from build123d import *

# Parameters (mm, degrees)
EXTRUDE_1_DEPTH = 95
SKETCH_3_W      = 60
SKETCH_3_H      = 60
EXTRUDE_3_DEPTH = 8.5
SKETCH_5_R      = 25
EXTRUDE_5_DEPTH = 3
SKETCH_7_R      = 7
EXTRUDE_6_DEPTH = 25
CHAMFER_1_SIZE  = 3


with BuildPart() as part:
    # 草图1 → 凸台-拉伸1 (new body)
    with BuildSketch(Plane.XY):
        with BuildLine():
            Line((7.5, 0), (52.5, 0))
            ThreePointArc((52.5, 0), (54.696699141, -5.303300859), (60, -7.5))
            Line((60, -7.5), (60, -52.5))
            ThreePointArc((60, -52.5), (54.696699141, -54.696699141), (52.5, -60))
            Line((52.5, -60), (7.5, -60))
            ThreePointArc((7.5, -60), (5.303300859, -54.696699141), (0, -52.5))
            Line((0, -52.5), (0, -7.5))
            ThreePointArc((0, -7.5), (5.303300859, -5.303300859), (7.5, 0))
        make_face()
    extrude(amount=EXTRUDE_1_DEPTH)

    # 草图3 → 凸台-拉伸3 (add)
    with BuildSketch(Plane(origin=(0, 0, 0), x_dir=(-1, 0, 0), z_dir=(0, 0, -1))):
        with Locations((-30, -30)):
            Rectangle(SKETCH_3_W, SKETCH_3_H)
    extrude(amount=EXTRUDE_3_DEPTH)

    # 草图5 → 凸台-拉伸5 (add)
    with BuildSketch(Plane(origin=(0, 0, -8.5), x_dir=(-1, 0, 0), z_dir=(0, 0, -1))):
        with Locations((-30, -30)):
            Circle(SKETCH_5_R)
    extrude(amount=EXTRUDE_5_DEPTH)

    # 草图7 → 凸台-拉伸6 (add)
    with BuildSketch(Plane(origin=(0, 0, -11.5), x_dir=(-1, 0, 0), z_dir=(0, 0, -1))):
        with Locations((-30, -30)):
            Circle(SKETCH_7_R)
    extrude(amount=EXTRUDE_6_DEPTH)

    # 倒角1
    chamfer_1_edges = [part.edges().sort_by_distance(p)[0] for p in [
        (0, -60, -4.25),
        (0, 0, -4.25),
        (60, 0, -4.25),
        (60, -60, -4.25),
    ]]
    chamfer(chamfer_1_edges, length=CHAMFER_1_SIZE)


solid = part.part
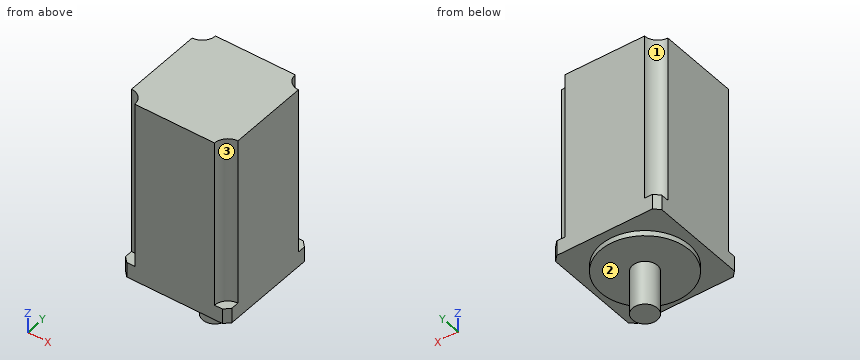
CAD build for the part. Positions are in the model's coordinates, mm. Face numbers are marked on the shaded views. A direction names the side the tool comes from. Coordinates: 2 decimals unless noted, no trailing zeros. Loops run counter-clockwise (first coordinate to the right, second up) from the corner with the lowest first, then second, coordinate; pieces in that order, holes last. Notation, with made-up numbers: (53.25, -4) -> (99.25, -4) arc R29 ccw to (99.25, 32) -> close; hole circle Ø1 at (37, -2.5). An arc over 180 degrees is marked (long way). One line per item, written item: value.
1. Drill centre lines: line 1 (Z direction, x = 23, y = -49); line 2 (Z direction, x = 45.5, y = -6); line 3 (Y direction, x = 56, z = 19). Where is each one in solid material? Low to high. Write a range as [from, to].
Answers:
line 1: z = [-11.5, 95]
line 2: z = [-8.5, 95]
line 3: y = [-53.66, -6.34]
2. Slice it at C-C on y = -30. Write the cut outline in (x, z), and give its area (3 significant figures).
Answers:
outline: (0, -8.5) -> (5, -8.5) -> (5, -11.5) -> (23, -11.5) -> (23, -36.5) -> (37, -36.5) -> (37, -11.5) -> (55, -11.5) -> (55, -8.5) -> (60, -8.5) -> (60, 95) -> (0, 95) -> close
area: 6,710 mm^2
3. Slice it at D-D on x = 11.5. Write the cut outline in (y, z).
Answers:
outline: (-60, -8.5) -> (-46.82, -8.5) -> (-46.82, -11.5) -> (-13.18, -11.5) -> (-13.18, -8.5) -> (0, -8.5) -> (0, 95) -> (-60, 95) -> close
4. Slice it at A-A on z = 44. Write the cut outline in (x, y), and give its area (3 significant figures).
Answers:
outline: (0, -52.5) arc R7.5 cw to (7.5, -60) -> (52.5, -60) arc R7.5 cw to (60, -52.5) -> (60, -7.5) arc R7.5 cw to (52.5, 0) -> (7.5, 0) arc R7.5 cw to (0, -7.5) -> close
area: 3,420 mm^2
5. Flat gauge pins, fed straight in: P1, Ø4, axis at x = 2, y = -2.5, coming from the +Z side; P2, Ø1.5, axis at x = 9.5, y = -12, coming from the -Z side; P3, Ø4, axis at x = 55, y = -56, coming from the +Z side; P4, Ø1, axis at x = 9.5, y = -23.5, coming from the -Z side. Where does each tip first touch, or does it go through?
Answers:
P1: stops at z = 0
P2: stops at z = -8.5
P3: stops at z = 95
P4: stops at z = -11.5
6. Slice it at B-B on x = 30. Write the cut outline in (y, z), and give its area (3 significant figures).
Answers:
outline: (-60, -8.5) -> (-55, -8.5) -> (-55, -11.5) -> (-37, -11.5) -> (-37, -36.5) -> (-23, -36.5) -> (-23, -11.5) -> (-5, -11.5) -> (-5, -8.5) -> (0, -8.5) -> (0, 95) -> (-60, 95) -> close
area: 6,710 mm^2
7. Which spindle directions (+Z, -Z, +X, -X, +Y, -Y) get a long thin tool onto all of the face, cutting with end or side? Do the marked faces 1, 2 and 3. Say none if no direction does.
Answers:
face 1: +Z, -X, +Y
face 2: -Z
face 3: +Z, +X, -Y
